Can you work these out from the model? Positions are in its coordinate system, mm. Face numbers are marked on the shaded views. A direction names the side the tool comes from. Coordinates: 2 decimals unless noted, no trailing zeros. Order: outer loops, then holes, each group sorted by start corner. A loop starts at its lowest first (then second) coordinate and runs counter-clockwise, first axis right, second up. Notation, with made-up numbers: (60.5, 25.25) -> (92.5, 25.25) arc R29 ccw to (92.5, 55.25) -> close; hole circle Ø11 at (17, 51.5). An arc over 180 degrees is marked (long way). Answer as a JSON object with one key per item and string values. Group by question number.
(1) I need wall thicknesses on line 1 (Y direction, x = 0, z = 3.55); line 2 (Y direction, x = 12.7, z = 16); line 3 (Y direction, x = 12.7, z = 4.75). Which ranges of each line are inside material? Lowest first, please.
(2) For pin 1 (5 mm diameter, centred on x = 12.7, y = 0, fed in from -Z); pin 2 (0.5 mm diameter, centred on x = 9, y = -7, fed in from +Z); pin 3 (1 mm diameter, centred on x = -2, y = -9.5, fed in from -Z); pin 4 (1.8 mm diameter, centred on x = 12.7, y = 0, fed in from +Z), each with a flat end and sliding along its axis, tell me the tip position at first contact or that it passes through.
(3) If we mould it in two halves opening along X, with no side actions, what happens to the marked faces 1, 2 and 3? For each: pulls with the +X half, pulls with the -X half, needs draft (parallel to the pull), parting line crosses it, or undercut.
(4) Which directions (+Z, -Z, +X, -X, +Y, -Y) give clear straight access to the entire face, cutting with the end or side of a thin tool? Please do the marked faces 4, 5, 6, 7 and 8.
(5) I want a section at A-A, the plane x = 5.5. List the corners of the cut face in (y, z) for me.
(6) I want a section at D-D, the plane y = 0. List the corners of the cut face in (x, z) for me.
(7) I want a section at B-B, the plane y = -11.35. List the corners of the cut face in (x, z) for me.
(8) I want a section at C-C, the plane z = 3.5. List the corners of the cut face in (x, y) for me.
from build123d import *

# Parameters (mm, degrees)
ESQUISSE1_W              = 40
ESQUISSE1_H              = 12.7
BOSS_EXTRU_1_DEPTH       = 23
CONG_1_R                 = 0.5
ESQUISSE2_R              = 1.5
ENL_V_MAT_EXTRU_1_DEPTH  = 24
ENL_V_MAT_EXTRU_2_DEPTH  = 5.5
ESQUISSE5_W              = 13
ESQUISSE5_H              = 8
ENL_V_MAT_EXTRU_3_DEPTH  = 18.5
BOSS_EXTRU_8_DEPTH       = 40
ESQUISSE16_R             = 4
ENL_V_MAT_EXTRU_10_DEPTH = 13
ESQUISSE18_R             = 4
ENL_V_MAT_EXTRU_11_DEPTH = 5
ESQUISSE19_R             = 1.5
ENL_V_MAT_EXTRU_12_DEPTH = 19


with BuildPart() as part:
    # Esquisse1 → Boss.-Extru.1 (new body)
    with BuildSketch(Plane.XY):
        Rectangle(ESQUISSE1_W, ESQUISSE1_H)
    extrude(amount=BOSS_EXTRU_1_DEPTH)

    # Congé1
    cong_1_edges = [part.edges().sort_by_distance(p)[0] for p in [
        (-20, 6.35, 11.5),
        (20, 6.35, 11.5),
    ]]
    fillet(cong_1_edges, radius=CONG_1_R)

    # Esquisse2 → Enlèv. mat.-Extru.1 (cut, through all)
    with BuildSketch(Plane.XY.offset(23)):
        with Locations((-12.7, 0)):
            Circle(ESQUISSE2_R)
        with Locations((12.7, 0)):
            Circle(ESQUISSE2_R)
    extrude(amount=-ENL_V_MAT_EXTRU_1_DEPTH, mode=Mode.SUBTRACT)

    # Esquisse4 → Enlèv. mat.-Extru.2 (cut)
    with BuildSketch(Plane(origin=(0, 0, 23), x_dir=(-1, 0, 0), z_dir=(0, 0, -1))):
        Polygon((-10, 6.35), (10, 6.35), (8.5, -6.85), (-8.5, -6.85), align=None)
    extrude(amount=ENL_V_MAT_EXTRU_2_DEPTH, mode=Mode.SUBTRACT)

    # Esquisse5 → Enlèv. mat.-Extru.3 (cut, through all)
    with BuildSketch(Plane.XY.offset(17.5)):
        with Locations((0, -0.25)):
            Rectangle(ESQUISSE5_W, ESQUISSE5_H)
    extrude(amount=-ENL_V_MAT_EXTRU_3_DEPTH, mode=Mode.SUBTRACT)

    # Esquisse17 → Boss.-Extru.8 (add)
    with BuildSketch(Plane.ZY.offset(20)):
        Polygon((8, -16.35), (0, -16.35), (0, -3.65), (23, -3.65), (23, -6.35), (14.45, -6.35), (14.45, -7.35), (11.55, -7.35), (11.55, -6.35), (8, -6.35), (8, -9.9), (9, -9.9), (9, -12.8), (8, -12.8), align=None)
    extrude(amount=-BOSS_EXTRU_8_DEPTH)

    # Esquisse16 → Enlèv. mat.-Extru.10 (cut)
    with BuildSketch(Plane(origin=(0, 0, 0), x_dir=(-1, 0, 0), z_dir=(0, 0, -1))):
        with Locations((-12.7, 0)):
            Circle(ESQUISSE16_R)
        with Locations((12.7, 0)):
            Circle(ESQUISSE16_R)
    extrude(amount=-ENL_V_MAT_EXTRU_10_DEPTH, mode=Mode.SUBTRACT)

    # Esquisse18 → Enlèv. mat.-Extru.11 (cut)
    with BuildSketch(Plane(origin=(0, 0, 0), x_dir=(-1, 0, 0), z_dir=(0, 0, -1))):
        with Locations((0, -11.35)):
            Circle(ESQUISSE18_R)
    extrude(amount=-ENL_V_MAT_EXTRU_11_DEPTH, mode=Mode.SUBTRACT)

    # Esquisse19 → Enlèv. mat.-Extru.12 (cut, through all)
    with BuildSketch(Plane(origin=(0, 0, 5), x_dir=(-1, 0, 0), z_dir=(0, 0, -1))):
        with Locations((0, -11.35)):
            Circle(ESQUISSE19_R)
    extrude(amount=-ENL_V_MAT_EXTRU_12_DEPTH, mode=Mode.SUBTRACT)


solid = part.part
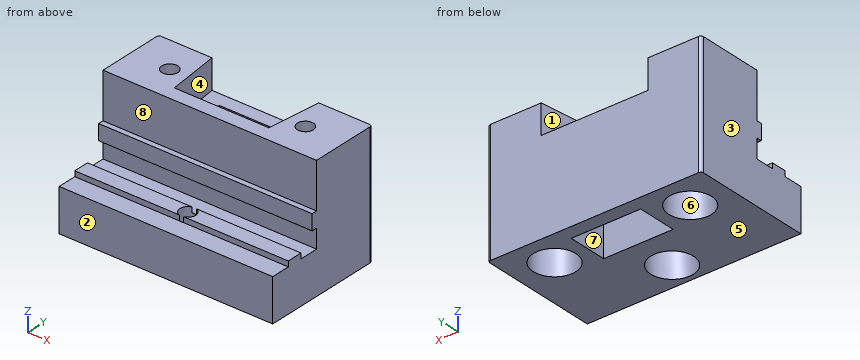
Computed values:
{
 "1": {"line 1": "y = -16.35 to -15.35, -7.35 to -3.65, 3.75 to 6.35", "line 2": "y = -6.35 to -1.5, 1.5 to 6.35", "line 3": "y = -16.35 to -4, 4 to 6.35"},
 "2": {"pin 1": "stops at z = 13", "pin 2": "stops at z = 14.45", "pin 3": "stops at z = 5", "pin 4": "passes through"},
 "3": {"face 1": "undercut", "face 2": "needs draft", "face 3": "pulls with the -X half"},
 "4": {"face 4": "+Z, +Y", "face 5": "-Z, +X, -X, +Y, -Y", "face 6": "-Z", "face 7": "+Z, -Z", "face 8": "+Z, +X, -X, -Y"},
 "5": {"outline": "(-16.35, 0) -> (-3.65, 0) -> (-3.65, 23) -> (-6.35, 23) -> (-6.35, 14.45) -> (-7.35, 14.45) -> (-7.35, 11.55) -> (-6.35, 11.55) -> (-6.35, 8) -> (-9.9, 8) -> (-9.9, 9) -> (-12.8, 9) -> (-12.8, 8) -> (-16.35, 8) -> close; (3.75, 0) -> (6.35, 0) -> (6.35, 17.5) -> (3.75, 17.5) -> close"},
 "6": {"outline": "(-20, 0) -> (-16.7, 0) -> (-16.7, 13) -> (-14.2, 13) -> (-14.2, 23) -> (-20, 23) -> close; (-11.2, 13) -> (-8.7, 13) -> (-8.7, 0) -> (-6.5, 0) -> (-6.5, 17.5) -> (-9.28, 17.5) -> (-9.28, 23) -> (-11.2, 23) -> close; (6.5, 0) -> (8.7, 0) -> (8.7, 13) -> (11.2, 13) -> (11.2, 23) -> (9.28, 23) -> (9.28, 17.5) -> (6.5, 17.5) -> close; (14.2, 13) -> (16.7, 13) -> (16.7, 0) -> (20, 0) -> (20, 23) -> (14.2, 23) -> close"},
 "7": {"outline": "(-20, 0) -> (-4, 0) -> (-4, 5) -> (-1.5, 5) -> (-1.5, 9) -> (-20, 9) -> close; (1.5, 5) -> (4, 5) -> (4, 0) -> (20, 0) -> (20, 9) -> (1.5, 9) -> close"},
 "8": {"outline": "(-20, -16.35) -> (20, -16.35) -> (20, 5.85) arc R0.5 ccw to (19.5, 6.35) -> (-19.5, 6.35) arc R0.5 ccw to (-20, 5.85) -> close; hole circle Ø8 at (-12.7, 0); hole (-6.5, -3.65) -> (6.5, -3.65) -> (6.5, 3.75) -> (-6.5, 3.75) -> close; hole circle Ø8 at (0, -11.35); hole circle Ø8 at (12.7, 0)"}
}
